Read the model definition and answer for the solid it produces. Units are mm, in the model's axes. A direction names the side the tool comes from. Give positions to 0.01 mm unless a question says otherwise; leave off trailing zeros. Order: outer loops, then holes, each group sorted by start corner. A loop starts at its lowest first (then second) coordinate and runs counter-clockwise, first axis right, second up. Notation, with made-up numbers: (68.25, 34.5) -> (120.25, 34.5) arc R16 ccw to (120.25, 63.5) -> close; hole circle Ø2 at (17.25, 81.25). An arc over 180 degrees is marked (long way). Use one line per item in the form item = value.
```python
from build123d import *

# Parameters (mm, degrees)
F0_R     = 109.5
F1_DEPTH = 50
F2_R     = 109.5
F2_R_2   = 106.5
F3_DEPTH = 40
F4_R     = 40
F5_DEPTH = 50.001


with BuildPart() as f1:
    # F0 (on Top) → F1 (new body)
    with BuildSketch(Plane.XY):
        Circle(F0_R)
    extrude(amount=F1_DEPTH)

    # F2 (on face) → F3 (cut)
    with BuildSketch(Plane(origin=(0, 0, 0), x_dir=(1, 0, 0), z_dir=(0, 0, -1))):
        Circle(F2_R)
        Circle(F2_R_2, mode=Mode.SUBTRACT)
    extrude(amount=-F3_DEPTH, mode=Mode.SUBTRACT)

    # F4 (on face) → F5 (cut, through all)
    with BuildSketch(Plane.XY.offset(50)):
        Circle(F4_R)
    extrude(amount=-F5_DEPTH, mode=Mode.SUBTRACT)


solid = f1.part
```
Item 1: The part is cut by section C-C on z = 45. Give the vertices of the cut face in (x, y).
Checks:
outline = circle Ø219 at (0, 0); hole circle Ø80 at (0, 0)
Item 2: Given pin 1 Ø1.5 at (y, z) = (73.5, 14) entering from -X; pin 2 Ø6 at (x, z) = (-52.5, 29.5) entering from +Y; pin 3 Ø1.5 at (y, z) = (42, 11) entering from +X, each flat-ended and moving along its own axis, determine where each tip first touches the part or whether it passes through.
Checks:
pin_1 = -77.78
pin_2 = 94.3
pin_3 = 98.19
Item 3: The part is cut by section D-D on x = -46. Give the vertices of the cut face in (y, z), and give its area (3 significant figures).
Checks:
outline = (-99.37, 40) -> (-96.05, 40) -> (-96.05, 0) -> (96.05, 0) -> (96.05, 40) -> (99.37, 40) -> (99.37, 50) -> (-99.37, 50) -> close
area = 9,670 mm²
Item 4: Determine the mould class of faces 1 (the cylindrical face through (-8.67, -39.05, 25.35)), 2 (the cylindrical face through (-23.737, -106.896, 44.93)), 3 (the flat face through (46, 1, 0)) for opening direction X: +X half, -X half, draft (parallel to the pull), parting line (faces both ways), or undercut.
Checks:
face_1 = undercut
face_2 = parting line
face_3 = draft
Item 5: Straight lines are drawn through the part: L1, parallel to Y at x = 0, z = 22.5; L2, parallel to X at y = -2.5, z = 29; L3, parallel to X at y = 29.5, z = 16. For each, find the intervals that lie inside material, in ascending order. Write a range as from..to.
Checks:
L1 = -106.5..-40, 40..106.5
L2 = -106.47..-39.92, 39.92..106.47
L3 = -102.33..-27.01, 27.01..102.33
Item 6: Which of the six approach directions +Z, -Z, +X, -X, +Y, -Y give full straight-line access (tool end or side, diameter ignored) to faces 4 (the flat face through (-2, -47, 50)), 5 (the cylindrical face through (-13.864, -105.594, 19.72))?
Checks:
face_4 = +Z, +X, -X, +Y, -Y
face_5 = -Z
Item 7: The part is cut by section A-A on y = 0. Give the vertices of the cut face in (x, z).
Checks:
outline = (-109.5, 40) -> (-106.5, 40) -> (-106.5, 0) -> (-40, 0) -> (-40, 50) -> (-109.5, 50) -> close; (40, 0) -> (106.5, 0) -> (106.5, 40) -> (109.5, 40) -> (109.5, 50) -> (40, 50) -> close
